Model file for the job. Use its own axes, mm. Give positions to 0.01 mm unless a question says otherwise; leave off trailing zeros. Order: outer loops, then holes, each group sorted by start corner. A loop starts at its lowest first (then second) coordinate and runs counter-clockwise, first axis right, second up. Notation, with made-up numbers: (-7.5, 28) -> (44.5, 28) arc R9 ccw to (44.5, 36) -> close; hole circle Ø9 at (81.5, 41). An arc over 180 degrees is marked (long way). Answer in a Markdown table with one row per item. Add a question column.
from build123d import *

# Parameters (mm, degrees)
SKETCH_1_W          = 170
SKETCH_1_H          = 20
EXTRUDE_1_DEPTH     = 5
EXTRUDE_2_DEPTH     = 5
FILLET_1_R          = 30
SKETCH_3_W          = 5
SKETCH_3_H          = 10
CUT_EXTRUDE_1_DEPTH = 10


with BuildPart() as part:
    # 스케치1 → 보스-돌출1 (new body)
    with BuildSketch(Plane(origin=(0, 0, 0), x_dir=(1, 0, 0), z_dir=(0, 1, 0))):
        with Locations((85, 10)):
            Rectangle(SKETCH_1_W, SKETCH_1_H)
    extrude(amount=EXTRUDE_1_DEPTH)

    # 스케치2 → 보스-돌출2 (add)
    with BuildSketch(Plane(origin=(0, 5, 0), x_dir=(1, 0, 0), z_dir=(0, 1, 0))):
        Polygon((0, 20), (55, 20), (0, 40), align=None)
        Polygon((115, 20), (170, 20), (170, 40), align=None)
    extrude(amount=-EXTRUDE_2_DEPTH)

    # 필렛1
    fillet_1_edges = [part.edges().sort_by_distance(p)[0] for p in [
        (55, 2.5, -20),
        (115, 2.5, -20),
    ]]
    fillet(fillet_1_edges, radius=FILLET_1_R)

    # 스케치3 → 컷-돌출1 (cut)
    with BuildSketch(Plane.XZ):
        with Locations((167.5, -5)):
            Rectangle(SKETCH_3_W, SKETCH_3_H)
        with Locations((167.5, -35)):
            Rectangle(SKETCH_3_W, SKETCH_3_H)
        with Locations((2.5, -35)):
            Rectangle(SKETCH_3_W, SKETCH_3_H)
        with Locations((2.5, -5)):
            Rectangle(SKETCH_3_W, SKETCH_3_H)
    extrude(amount=-CUT_EXTRUDE_1_DEPTH, mode=Mode.SUBTRACT)


solid = part.part
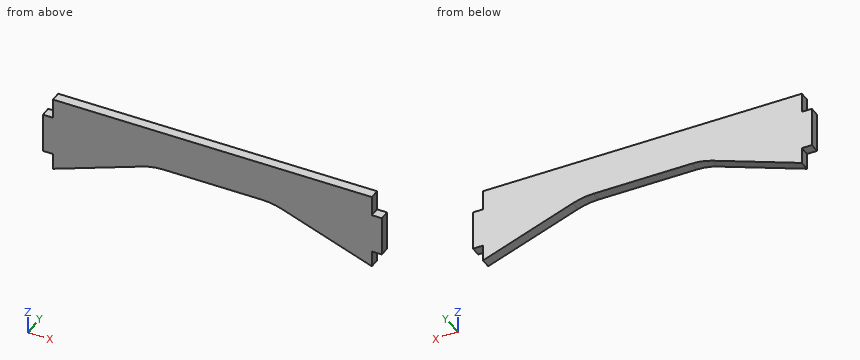
Item 1: Saw through at B-B on y = 3.1. List the corners of the cut face in (x, z), plus the area to 3 significant figures.
Item 2: Pin check, flat tips, straight feed: pin 1 Ø2.5 at (y, z) = (3, -6.5) entering from -X; pin 2 Ø2.5 at (x, y) = (167, 1.5) entering from +Z; pin 3 Ø2.5 at (y, z) = (3.5, -34.5) entering from +X. Stop position of each tip, or through.
Item 3: Wall check: line 1 (X direction, y = 0.35, z = -2); line 2 (Z direction, x = 81, y = 0.3); line 3 (Z direction, x = 136, y = 3.7). Give the ranges that are in metal, low to high.
Item 4: Saw through at D-D on x = 92.5. List the corners of the cut face in (y, z), plus the area to 3 significant figures.
Item 5: Saw through at C-C on z = -27.5. List the corners of the cut face in (x, y) (3 decimals), plus the area to 3 significant figures.
Item 6: Saw through at A-A on z = -35. List the corners of the cut face in (x, y).
Evaluation:
| question | item | result |
|---|---|---|
| 1 | outline | (0, -30) -> (5, -30) -> (5, -38.18) -> (50.03, -21.81) arc R30 cw to (60.29, -20) -> (109.71, -20) arc R30 cw to (119.97, -21.81) -> (165, -38.18) -> (165, -30) -> (170, -30) -> (170, -10) -> (165, -10) -> (165, 0) -> (5, 0) -> (5, -10) -> (0, -10) -> close |
| 1 | area | 4,310 mm2 |
| 2 | pin 1 | stops at x = 5 |
| 2 | pin 2 | stops at z = -10 |
| 2 | pin 3 | stops at x = 165 |
| 3 | line 1 | x = 5 to 165 |
| 3 | line 2 | z = -20 to 0 |
| 3 | line 3 | z = -27.64 to 0 |
| 4 | outline | (0, -20) -> (5, -20) -> (5, 0) -> (0, 0) -> close |
| 4 | area | 100 mm2 |
| 5 | outline | (0, 0) -> (34.375, 0) -> (34.375, 5) -> (0, 5) -> close; (135.625, 0) -> (170, 0) -> (170, 5) -> (135.625, 5) -> close |
| 5 | area | 344 mm2 |
| 6 | outline | (5, 0) -> (13.75, 0) -> (13.75, 5) -> (5, 5) -> close; (156.25, 0) -> (165, 0) -> (165, 5) -> (156.25, 5) -> close |
